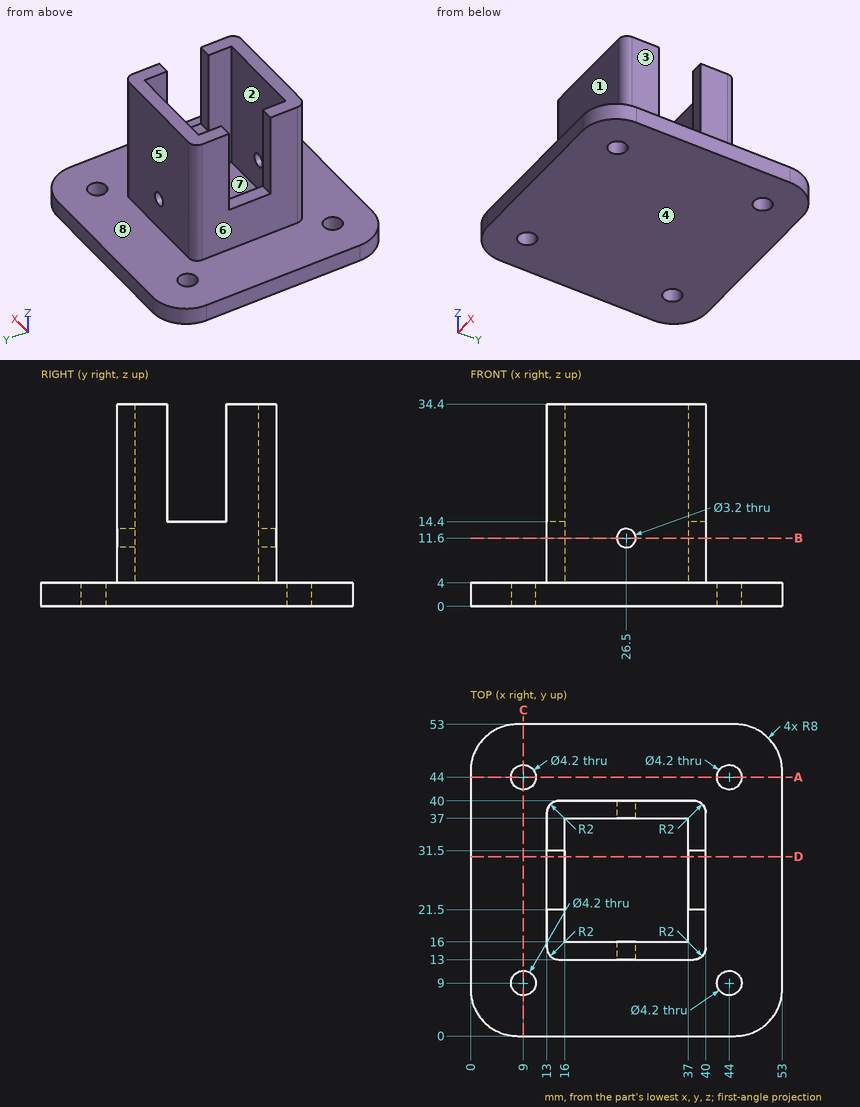
Check sheet for the drawn part. Datum: minimum x, y, z corner. Units: mm. A direction names the side the tool comes from. Round coordinates to 2 decimals unless told otherwise and drop trailing zeros. Order: outer loops, then holes, each group sorted by start corner. A loop starts at its lowest first (then second) coordinate and runs counter-clockwise, first axis right, second up. Notation, with made-up numbers: M 24.25,20 L 81.25,20 A17 cw 81.25,36 Z; hole C 33,42.5 d7. An arc over 180 degrees is marked long. Answer in a Markdown table with one row per item.
(1) Section check B-B on z = 11.6. Record the boundary of the cut face in (x, y), plus the area to 3 significant figures.
Findings:
| item | result |
|---|---|
| outline | M 13,15 A2 ccw 15,13 L 24.9,13 L 24.9,16 L 16,16 L 16,37 L 24.9,37 L 24.9,40 L 15,40 A2 ccw 13,38 Z; M 28.1,13 L 38,13 A2 ccw 40,15 L 40,38 A2 ccw 38,40 L 28.1,40 L 28.1,37 L 37,37 L 37,16 L 28.1,16 Z |
| area | 265 mm^2 |
(2) Draft check along X on the marked faces 6, 7 and 8. Enter one of: +X half, -X half, draft (parallel to the pull), parting line (faces both ways), or undercut.
Findings:
| item | result |
|---|---|
| face 6 | -X half |
| face 7 | undercut |
| face 8 | draft |
(3) Section check D-D on y = 30.5. Record the boundary of the cut face in (x, z), plus the area to 3 significant figures.
Findings:
| item | result |
|---|---|
| outline | M 0,0 L 53,0 L 53,4 L 40,4 L 40,14.4 L 37,14.4 L 37,4 L 16,4 L 16,14.4 L 13,14.4 L 13,4 L 0,4 Z |
| area | 274 mm^2 |
(4) Set-up check for the marked faces 1, 2, 3, 4 and 5: record each of +Z, -Z, +X, -X, +Y, -Y from which the full face is reachable in a straight line by a thin tool's end or side.
Findings:
| item | result |
|---|---|
| face 1 | +Z, +X, -X, -Y |
| face 2 | +Z |
| face 3 | +Z, +X, +Y, -Y |
| face 4 | -Z, +X, -X, +Y, -Y |
| face 5 | +Z, +X, -X, +Y |
(5) Material ranges on line 1 along Y through (x, z) = (15.5, 20); line 2 along Y through (x, z) = (43, 2); line 3 along Z through (x, y) = (15.5, 49), recorded low to high. Write a range as from..to.
Findings:
| item | result |
|---|---|
| line 1 | y = 13..21.5, 31.5..40 |
| line 2 | y = 0..7.15, 10.85..42.15, 45.85..53 |
| line 3 | z = 0..4 |
(6) Section check A-A on y = 44. Record the boundary of the cut face in (x, z), plus the area to 3 significant figures.
Findings:
| item | result |
|---|---|
| outline | M 0,0 L 6.9,0 L 6.9,4 L 0,4 Z; M 11.1,0 L 41.9,0 L 41.9,4 L 11.1,4 Z; M 46.1,0 L 53,0 L 53,4 L 46.1,4 Z |
| area | 178 mm^2 |
(7) Gauge pin test, flat ends, axial feed: pin 1 (1 mm diameter, centred on x = 16, z = 21.5, fed in from -Y); pin 2 (11.5 mm diameter, centred on x = 30.5, z = 12, fed in from +Y); pin 3 (5 mm diameter, centred on y = 36.5, z = 20.5, fed in from +X); pin 4 (1 mm diameter, centred on x = 47, y = 5.5, fed in from -Z). Record the tip position at first contact, or that the pin passes through.
Findings:
| item | result |
|---|---|
| pin 1 | stops at y = 13 |
| pin 2 | stops at y = 40 |
| pin 3 | stops at x = 40 |
| pin 4 | stops at z = 0 |
